from build123d import *

# Parameters (mm, degrees)
SKETCH1_W                    = 36.195
SKETCH1_H                    = 1.5875
F_36_0_1065_DIAMETER_HOLE1_D = 2.7051
CIRPATTERN1_COUNT            = 12


with BuildPart() as part:
    # Sketch1 → Revolve1 (revolve)
    with BuildSketch(Plane.XY):
        with Locations((-27.6225, 0.79375)):
            Rectangle(SKETCH1_W, SKETCH1_H)
    revolve(axis=Axis((0, 55, 0), (0, -1, 0)))

    # #36 (0.1065) Diameter Hole1 (through all)
    with Locations(Plane(origin=(0, 1.5875, 0), x_dir=(1, 0, 0), z_dir=(0, 1, 0))):
        with Locations((-42.700575, 0)):
            f_36_0_1065_diameter_hole1 = Hole(F_36_0_1065_DIAMETER_HOLE1_D / 2)

    # CirPattern1: #36 (0.1065) Diameter Hole1 ×12 about axis
    cirpattern1_axis = Axis((0, 0, 0), (0, 1, 0))
    for i in range(1, CIRPATTERN1_COUNT):
        add(f_36_0_1065_diameter_hole1.rotate(cirpattern1_axis, i * 360 / CIRPATTERN1_COUNT), mode=Mode.SUBTRACT)


solid = part.part
Verification items for the finished model (mm, model axes). Coordinates: 2 decimals unless noted, no trailing zeros. Loops run counter-clockwise (first coordinate to the right, second up) from the corner with the lowest first, then second, coordinate; pieces in that order, holes last. Notation, with made-up numbers: M -7.75,-35.75 L -2.75,-35.75 A20 cw -2.75,-25.75 Z; hole C 3.5,45 d8. An arc over 180 degrees is marked long. One line per item, written item: value.
1. Material ranges on line 1 along Z through (x, y) = (-1, 0.15); line 2 along Z through (x, y) = (8, 0.45); line 3 along X through (y, z) = (0.4, -19.5), recorded low to high. Write a range as from..to.
Answers follow:
line 1: -45.71..-43.61, -41.79..-9.47, 9.47..41.79, 43.61..45.71
line 2: -45.01..-5.17, 5.17..45.01
line 3: -41.35..41.35
2. Gauge pin test, flat end, axial feed: P1, Ø1.6, axis at x = -36.98, z = 21.35, coming from the +Y side. Record the tip position at first contact, or that the pin passes through.
Answers follow:
P1: through
3. Section check C-C on y = 1.3. Give the number of separate pieces and of enclosed holes in the cut face, plus the area to 3 significant figures.
Answers follow:
separate pieces: 1
enclosed holes: 13
area: 6,210 mm^2
4. Section check A-A on x = 0. Record the cut outline in (y, z) (1 decimal).
Answers follow:
outline: M 0,-45.7 L 1.6,-45.7 L 1.6,-44.1 L 0,-44.1 Z; M 0,-41.3 L 1.6,-41.3 L 1.6,-9.5 L 0,-9.5 Z; M 0,9.5 L 1.6,9.5 L 1.6,41.3 L 0,41.3 Z; M 0,44.1 L 1.6,44.1 L 1.6,45.7 L 0,45.7 Z
5. Section check D-D on x = 18.5. Record the cut outline in (y, z).
Answers follow:
outline: M 0,-41.81 L 1.59,-41.81 L 1.59,41.81 L 0,41.81 Z
6. Mould release check, pull along X, two halves, no side actions. Record for faces 1 (the cylindrical face through (-41.7, 0.78, -0.91)), 2 (the cylindrical face through (-43.61, 0.8, -13.73)), 3 (the flat face through (1, 0, 10)): pulls with the +X half, pulls with the -X half, needs draft (parallel to the pull), parting line crosses it, or undercut.
Answers follow:
face 1: undercut
face 2: parting line crosses it
face 3: needs draft
7. Section check B-B on z = 0. Record the cut outline in (x, y) (1 decimal).
Answers follow:
outline: M -45.7,0 L -44.1,0 L -44.1,1.6 L -45.7,1.6 Z; M -41.3,0 L -9.5,0 L -9.5,1.6 L -41.3,1.6 Z; M 9.5,0 L 41.3,0 L 41.3,1.6 L 9.5,1.6 Z; M 44.1,0 L 45.7,0 L 45.7,1.6 L 44.1,1.6 Z
